Design review of the part shown in the three views and the two pictorial views. Dimensions are in mm from the part's minimum x, y and z. A direction names the side the tool comes from. Round coordinates to 2 decimals unless told otherwise and drop trailing zeros. Loops run counter-clockwise (first coordinate to the right, second up) from the corner with the lowest first, then second, coordinate; pieces in that order, holes last. Notation, with made-up numbers: (-33.75, 60.25) - (15.25, 60.25) arc R30 cw to (15.25, 86.25) - close; hole circle Ø9 at (38.25, 58.25). An arc over 180 degrees is marked (long way). Return JSON: item names as keys, results as strings. Group by question number.
(1) We need section A-A, the plane z = 101.6. Write out the cut boundary in (x, y).
(2) We need section D-D, the plane x = 57.15. Write out the cut boundary in (y, z).
(3) We need section B-B, the plane y = 87.5. Write out the cut boundary in (x, z).
(4) Clearance check with flat-ended pins moving along their axes: pin 1 (10 mm diameter, centred on y = 27.5, z = 59, fed in from +X); pin 2 (13.5 mm diameter, centred on y = 70, z = 13, fed in from +X); pin 3 (12 mm diameter, centred on x = 136, y = 46.5, fed in from -Z). State where each tip first meets the part, or that it passes through.
(5) The part is to be moulded in two halves that separate along Z. For the marked faces 4, 5 and 6, say which applies: pulls with the +Z half, pulls with the -Z half, needs draft (parallel to the pull), parting line crosses it, or undercut.
(6) For the marked faces 1, 2 and 3, list the 3-axis set-ups (+Z, -Z, +X, -X, +Y, -Y) from which the entire face can be reached by the end or side of a thin tool; tool diameter is ignored.
(7) We need section C-C, the plane z = 31.5. Write out the cut boundary in (x, y), and give its area (3 significant figures).
(8) Wall thickness on L1, parallel to Z at x = 107.95, y = 111.5; L2, parallel to Y at x = 134, z = 94.5: over which ranges is each line inside the solid? List them lowest first. Write a range as [from, to].
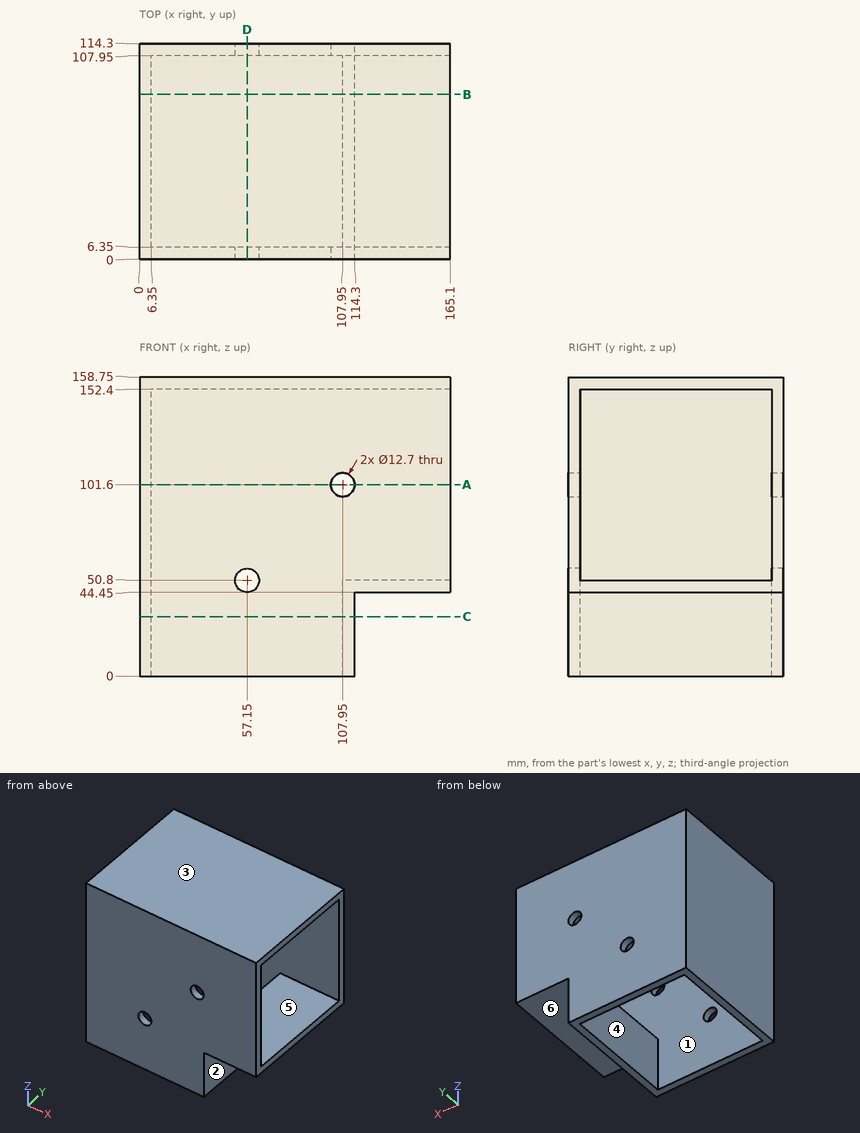
Solutions:
{
 "1": {"outline": "(0, 0) - (101.6, 0) - (101.6, 6.35) - (6.35, 6.35) - (6.35, 107.95) - (101.6, 107.95) - (101.6, 114.3) - (0, 114.3) - close; (114.3, 0) - (165.1, 0) - (165.1, 6.35) - (114.3, 6.35) - close; (114.3, 107.95) - (165.1, 107.95) - (165.1, 114.3) - (114.3, 114.3) - close"},
 "2": {"outline": "(0, 0) - (6.35, 0) - (6.35, 44.45) - (0, 44.45) - close; (0, 57.15) - (6.35, 57.15) - (6.35, 152.4) - (107.95, 152.4) - (107.95, 57.15) - (114.3, 57.15) - (114.3, 158.75) - (0, 158.75) - close; (107.95, 0) - (114.3, 0) - (114.3, 44.45) - (107.95, 44.45) - close"},
 "3": {"outline": "(0, 0) - (6.35, 0) - (6.35, 152.4) - (165.1, 152.4) - (165.1, 158.75) - (0, 158.75) - close; (107.95, 0) - (114.3, 0) - (114.3, 44.45) - (165.1, 44.45) - (165.1, 50.8) - (107.95, 50.8) - close"},
 "4": {"pin 1": "x = 6.35", "pin 2": "x = 114.3", "pin 3": "z = 44.45"},
 "5": {"face 4": "needs draft", "face 5": "undercut", "face 6": "pulls with the -Z half"},
 "6": {"face 1": "none", "face 2": "-Z, +X, +Y, -Y", "face 3": "+Z, +X, -X, +Y, -Y"},
 "7": {"outline": "(0, 0) - (114.3, 0) - (114.3, 114.3) - (0, 114.3) - close; hole (6.35, 6.35) - (107.95, 6.35) - (107.95, 107.95) - (6.35, 107.95) - close", "area": "2,740 mm^2"},
 "8": {"L1": "[0, 95.25], [107.95, 158.75]", "L2": "[0, 6.35], [107.95, 114.3]"}
}
